For this review, take the finished solid that the model builds, in its own axes (mm). A direction names the side the tool comes from. Give positions to 0.01 mm unless a question says otherwise; leave off trailing zeros. Write each loop counter-clockwise with the first axis right and the second up, starting at its lowest first coordinate (ties: lowest second). Pieces come first, ordered by that corner, then holes.
Q1. Machinability: for faces 1 (the flat face through (15, 4, -114)), 2 (the cylindrical face through (55, -13, -14)), 3 (the flat face through (-15, 4, -114)), which of the approach directions +Z, -Z, +X, -X, +Y, -Y give a long, thin tool a straight path to every point of the face, cutting with its end or side? Answer none if there is none.
Q2. We need section C-C (z = -187.5). Write out the cut boundary in (x, y), then the cut area to 3 significant figures.
Q3. We need section A-A (x = 0). Write out the cut boundary in (y, z), then the cut area to 3 significant figures.
Q4. Insertion check: P1, Ø3, axis at x = 62.5, z = -0.5, coming from the +Y side; P2, Ø1.2, axis at x = -64, z = -0.5, coming from the +Y side; P3, Ø7.5, axis at x = 0, y = 30, coming from the -Z side; P4, Ø13.5, axis at y = 30, z = 0, coming from the +X side. Each pin has a flat end and moves straight along its axis. Give the tip position at first contact, or say it passes through.
Q5. Mouldability with a two-part tool opening along Z and no side actions: class faces 4 (the cylindrical face through (-0.187, 25.754, -206.25)), 5 (the cylindrical face through (78, 25, -14)), 6 (the cylindrical face through (14, 13, -107)) as released by +Z, released by -Z, zero draft, split by the parting line, or undercut.
Q6. We need section B-B (x = 84). Write out the cut boundary in (y, z), then the cut area to 3 significant figures.
Q7. For line 1 (Z direction, x = 6, y = 10); line 2 (Z direction, x = 6, y = 11); line 3 (X direction, y = 13, z = 0), list the stretches that pass through material, from the lowest coordinate up.
Autodesk Inventor part; units mm, degrees
ref_plane "YZ Plane" through (0, 0, 0) normal (1, 0, 0) x (0, 1, 0)
ref_plane "XZ Plane" through (0, 0, 0) normal (0, 1, 0) x (-1, 0, 0)
ref_plane "XY Plane" through (0, 0, 0) normal (0, 0, 1) x (1, 0, 0)
sketch "Sketch1" plane through (0, 0, 0) normal (0, 1, 0) x (-1, 0, 0)
  line L0 (96, 15) -> (-96, 15)
  line L1 (-96, 15) -> (-96, -15)
  line L2 (96, -15) -> (96, 15)
  line L3 (96, 15) -> (-96, -15) construction
  line L4 (-96, 15) -> (96, -15) construction
  line L5 (0, 0) -> (0, -223) construction
  line L6 (15, -211.066) -> (15, -15)
  line L7 (-96, -15) -> (-15, -15)
  line L8 (15, -15) -> (96, -15)
  line L9 (-15, -211.066) -> (-15, -15)
  line L10 (15, -211.066) -> (-15, -211.066)
  dimension "d0" = 192
  dimension "d1" = 30
  dimension "d2" = 196.066
  dimension "d3" = 15
extrude "Extrusion1" add sketch "Sketch1" along normal mid plane 30
sketch "Sketch2" plane through (0, 15, 0) normal (0, 1, 0) x (1, 0, 0)
  line L0 (15, 15) -> (96, 15)
  line L1 (96, -15) -> (-96, -15)
  line L2 (96, 15) -> (76, 15)
  line L3 (76, 15) -> (76, -15)
  line L4 (76, -15) -> (96, -15)
  line L5 (96, -15) -> (96, 15)
  line L6 (15, 211.066) -> (15, 15)
  line L7 (-15, 15) -> (-15, 211.066)
  line L8 (15, 211.066) -> (-15, 211.066)
  line L9 (-15, 211.066) -> (-15, 191.066)
  line L10 (-15, 191.066) -> (15, 191.066)
  line L11 (15, 191.066) -> (15, 211.066)
  line L12 (-96, 15) -> (-15, 15)
  line L13 (-96, -15) -> (-76, -15)
  line L14 (-76, -15) -> (-76, 15)
  line L15 (-76, 15) -> (-96, 15)
  line L16 (-96, 15) -> (-96, -15)
  point P0 (0, 0)
  point P1 (-15, 211.066)
  point P2 (15, 191.066)
  point P3 (76, 15)
  point P4 (-76, -15)
  dimension "d6" = 20
  dimension "d7" = 20
  dimension "d8" = 20
extrude "Extrusion2" add sketch "Sketch2" along normal blind 30 contours L0 L5 L1 L3 | L10 L7 L8 L6 | L1 L16 L12 L14
fillet "Fillet1" radius 5 38 edges at (15, 0, -15) (-15, 0, -15) (15, -15, -113.033) (55.5, -15, -15) (-55.5, -15, -15) (0, -15, 15) (96, -15, 0) (96, 15, -15) (96, 15, 15) (96, 45, 0) (-96, 15, 15) (-96, -15, 0) (-96, 15, -15) (-96, 45, 0) (-15, 15, -211.066) (15, 15, -211.066) (0, 45, -211.066) (0, 45, -191.066) (0, 15, 15) (-76, 45, 0) (-86, 45, 15) (-86, 45, -15) (86, 45, -15) (86, 45, 15) (76, 45, 0) (15, 45, -201.066) (-15, 45, -201.066) (76, 30, 15) (76, 30, -15) (-76, 30, 15) (-76, 30, -15) (15, 30, -191.066) (-15, 30, -191.066) (-15, -15, -113.033) (-15, 15, -103.033) (15, 15, -103.033) (45.5, 15, -15) (-45.5, 15, -15)
sketch "Sketch3" plane through (0, 15, 0) normal (0, 1, 0) x (1, 0, 0)
  line L0 (-76, 10) -> (-76, -10)
  line L1 (-81, -15) -> (81, -15)
  line L2 (76, -10) -> (76, 10)
  line L3 (-15, 196.066) -> (-15, 20)
  line L4 (-10, 191.066) -> (10, 191.066)
  line L5 (10, 191.066) -> (-10, 191.066)
  line L6 (15, 20) -> (15, 196.066)
  point P0 (0, 0)
  point P1 (-63.5, 0)
  point P2 (63.5, 0)
  point P3 (6, 176.066)
  point P4 (-6, 176.066)
  point P5 (6, 91.066)
  point P6 (-6, 91.066)
  point P7 (-6, 75)
  point P8 (6, 75)
  dimension "d19" = 12.5
  dimension "d20" = 15
  dimension "d21" = 15
  dimension "d22" = 12.5
  dimension "d23" = 90
  dimension "d24" = 90
  dimension "d25" = 9
  dimension "d26" = 100
  dimension "d27" = 9
  dimension "d28" = 100
  dimension "d29" = 9
  dimension "d30" = 9
  dimension "d58" = 15
  dimension "d59" = 15
  dimension "d60" = 9
  dimension "d61" = 9
hole "Hole1" at (-63.5, 15, 0) at (63.5, 15, 0) at (-6, 15, -91.066) at (6, 15, -91.066) at (6, 15, -75) at (-6, 15, -75) at (6, 15, -176.066) at (-6, 15, -176.066) direction (0, -1, 0) diameter 4 depth 7 countersink diameter 4.2 countersink angle 90
sketch "Sketch7" plane through (76, 15, -10) normal (-1, 0, 0) x (0, 0, 1)
  line L0 (-5, 25) -> (-5, -5)
  line L1 (20, 30) -> (0, 30)
  point P0 (10, -15)
  point P1 (10, 15)
  dimension "d83" = 15
  dimension "d84" = 15
hole "Hole5" at (76, 30, 0) direction (1, 0, 0) diameter 9.8 depth 10.5 countersink diameter 10.5 countersink angle 90
sketch "Sketch8" plane through (-76, 15, 10) normal (1, 0, 0) x (0, 0, -1)
  line L0 (20, 30) -> (0, 30)
  line L1 (25, -5) -> (25, 25)
  point P0 (10, -15)
  point P1 (10, 15)
  dimension "d85" = 15
  dimension "d86" = 15
hole "Hole6" at (-76, 30, 0) direction (-1, 0, 0) diameter 9.8 depth 10.5 countersink diameter 10.5 countersink angle 90
sketch "Sketch9" plane through (-10, 15, -191.066) normal (0, 0, 1) x (1, 0, 0)
  line L0 (-5, 25) -> (-5, -5)
  line L1 (20, 30) -> (0, 30)
  point P0 (10, -15)
  point P1 (10, 15)
  dimension "d87" = 15
  dimension "d88" = 15
hole "Hole7" at (0, 30, -191.066) direction (0, 0, -1) diameter 9.8 depth 10.5 countersink diameter 10.5 countersink angle 90
sketch "Sketch10" plane through (96, -10, -10) normal (1, 0, 0) x (0, 0, -1)
  line L0 (0, 55) -> (-20, 55)
  line L1 (5, 0) -> (5, 50)
  point P0 (-10, 10)
  point P1 (-10, 40)
  dimension "d89" = 15
  dimension "d90" = 15
hole "Hole8" at (96, 30, 0) direction (-1, 0, 0) diameter 8.5 end through all
sketch "Sketch11" plane through (10, 40, -211.066) normal (0, 0, -1) x (-1, 0, 0)
  line L0 (20, 5) -> (0, 5)
  line L1 (25, -50) -> (25, 0)
  point P0 (10, -40)
  point P1 (10, -10)
  dimension "d98" = 15
  dimension "d99" = 15
hole "Hole9" at (0, 30, -211.066) direction (0, 0, 1) diameter 8.5 end through all
properties part number "Tcalev2"
Computed:
1. face 1: -Z, +X, +Y, -Y
1. face 2: -Z, +X, -Y
1. face 3: -Z, -X, +Y, -Y
2. outline: (-15, -10) arc R5 ccw to (-10, -15) - (10, -15) arc R5 ccw to (15, -10) - (15, 10) arc R5 ccw to (10, 15) - (-10, 15) arc R5 ccw to (-15, 10) - close
2. area: 879 mm2
3. outline: (-15, -211.07) - (25.75, -211.07) - (25.75, -201.57) - (25.1, -201.57) - (25.1, -191.42) - (24.75, -191.07) - (15, -191.07) - (15, 10) arc R5 ccw to (10, 15) - (-10, 15) arc R5 ccw to (-15, 10) - close; (34.25, -211.07) - (40, -211.07) arc R5 ccw to (45, -206.07) - (45, -196.07) arc R5 ccw to (40, -191.07) - (35.25, -191.07) - (34.9, -191.42) - (34.9, -201.57) - (34.25, -201.57) - close
3. area: 7,180 mm2
4. P1: stops at y = 15
4. P2: stops at y = 8
4. P3: passes through
4. P4: stops at x = 96
5. face 4: zero draft
5. face 5: released by -Z
5. face 6: undercut
6. outline: (-15, -10) arc R5 ccw to (-10, -15) - (40, -15) arc R5 ccw to (45, -10) - (45, 10) arc R5 ccw to (40, 15) - (-10, 15) arc R5 ccw to (-15, 10) - close; hole circle Ø9.8 at (30, 0)
6. area: 1,700 mm2
7. line 1: z = -211.07 to -178.07, -174.07 to -93.07, -89.07 to -77, -73 to 15
7. line 2: z = -211.07 to -178.07, -174.07 to -93.07, -89.07 to -77, -73 to 14.9
7. line 3: x = -96 to -65.5, -61.5 to 61.5, 65.5 to 96
